Part model, mm, in its own coordinate system. A direction names the side the tool comes from. Give positions to 0.01 mm unless a question says otherwise; leave off trailing zeros. Loops run counter-clockwise (first coordinate to the right, second up) from the corner with the lowest first, then second, coordinate; pieces in that order, holes last. Notation, with made-up numbers: M 12,42 L 26,42 A27 cw 26,61 Z; hole C 20,-17.75 d8. An arc over 180 degrees is marked long. Answer in a Markdown table with one row per item.
from build123d import *

# Parameters (mm, degrees)
SKETCH1_R           = 2.5
BOSS_EXTRUDE1_DEPTH = 2.5


with BuildPart() as part:
    # Sketch1 → Boss-Extrude1 (new body)
    with BuildSketch(Plane(origin=(0, 0, -1.25), x_dir=(-1, 0, 0), z_dir=(0, 0, -1))):
        with BuildLine():
            Line((44.196, 6.35), (13.62993597, 36.91606403))
            ThreePointArc((13.62993597, 36.91606403), (12.941682484, 37.946108163), (12.7, 39.161128061))
            Line((12.7, 39.161128061), (12.7, 50.546))
            Line((12.7, 50.546), (6.35, 56.896))
            Line((6.35, 56.896), (-6.35, 56.896))
            Line((-6.35, 56.896), (-12.7, 50.546))
            Line((-12.7, 50.546), (-12.7, 39.161128061))
            ThreePointArc((-12.7, 39.161128061), (-12.941682484, 37.946108163), (-13.62993597, 36.91606403))
            Line((-13.62993597, 36.91606403), (-44.196, 6.35))
            Line((-44.196, 6.35), (-44.196, -6.35))
            Line((-44.196, -6.35), (-37.846, -12.7))
            Line((-37.846, -12.7), (37.846, -12.7))
            Line((37.846, -12.7), (44.196, -6.35))
            Line((44.196, -6.35), (44.196, 6.35))
        make_face()
        with Locations((0, 50.8)):
            Circle(SKETCH1_R, mode=Mode.SUBTRACT)
        with Locations((0, 38.1)):
            Circle(SKETCH1_R, mode=Mode.SUBTRACT)
        with Locations((-38.1, 0)):
            Circle(SKETCH1_R, mode=Mode.SUBTRACT)
        with Locations((-25.4, 0)):
            Circle(SKETCH1_R, mode=Mode.SUBTRACT)
        with Locations((-12.7, 0)):
            Circle(SKETCH1_R, mode=Mode.SUBTRACT)
        Circle(SKETCH1_R, mode=Mode.SUBTRACT)
        with Locations((12.7, 0)):
            Circle(SKETCH1_R, mode=Mode.SUBTRACT)
        with Locations((38.1, 0)):
            Circle(SKETCH1_R, mode=Mode.SUBTRACT)
        with Locations((25.4, 0)):
            Circle(SKETCH1_R, mode=Mode.SUBTRACT)
        with Locations((0, 12.7)):
            Circle(SKETCH1_R, mode=Mode.SUBTRACT)
        with Locations((0, 25.4)):
            Circle(SKETCH1_R, mode=Mode.SUBTRACT)
        with Locations((25.4, 12.7)):
            Circle(SKETCH1_R, mode=Mode.SUBTRACT)
        with Locations((12.7, 12.7)):
            Circle(SKETCH1_R, mode=Mode.SUBTRACT)
        with Locations((12.7, 25.4)):
            Circle(SKETCH1_R, mode=Mode.SUBTRACT)
        with Locations((-12.7, 12.7)):
            Circle(SKETCH1_R, mode=Mode.SUBTRACT)
        with Locations((-12.7, 25.4)):
            Circle(SKETCH1_R, mode=Mode.SUBTRACT)
        with Locations((-25.4, 12.7)):
            Circle(SKETCH1_R, mode=Mode.SUBTRACT)
    extrude(amount=-BOSS_EXTRUDE1_DEPTH)


solid = part.part
(1) Saw through at B-B (y = -1.5). Give the number of separate pieces and of enclosed holes in the cut face, plus the area to 3 significant figures.
Recorded:
| item | result |
|---|---|
| separate pieces | 8 |
| enclosed holes | 0 |
| area | 151 mm^2 |
(2) Saw through at D-D (y = 38.1). Write the cut outline in (x, z), plus the area to 3 significant figures.
Recorded:
| item | result |
|---|---|
| outline | M -12.88,-1.25 L -2.5,-1.25 L -2.5,1.25 L -12.88,1.25 Z; M 2.5,-1.25 L 12.88,-1.25 L 12.88,1.25 L 2.5,1.25 Z |
| area | 51.9 mm^2 |
(3) Saw through at A-A (y = 12.7). Write the cut outline in (x, z), plus the area to 3 significant figures.
Recorded:
| item | result |
|---|---|
| outline | M -37.85,-1.25 L -27.9,-1.25 L -27.9,1.25 L -37.85,1.25 Z; M -22.9,-1.25 L -15.2,-1.25 L -15.2,1.25 L -22.9,1.25 Z; M -10.2,-1.25 L -2.5,-1.25 L -2.5,1.25 L -10.2,1.25 Z; M 2.5,-1.25 L 10.2,-1.25 L 10.2,1.25 L 2.5,1.25 Z; M 15.2,-1.25 L 22.9,-1.25 L 22.9,1.25 L 15.2,1.25 Z; M 27.9,-1.25 L 37.85,-1.25 L 37.85,1.25 L 27.9,1.25 Z |
| area | 127 mm^2 |
(4) Pull direction X, two halves, no side cores. Call faces 3 (the face through (44.196, 0, 0)), 4 (the face through (1, 7, -1.25)), 5 (the face through (15.2, 0.1, 0)): +X half, -X half, draft (parallel to the pull), parting line (faces both ways), or undercut.
Recorded:
| item | result |
|---|---|
| face 3 | +X half |
| face 4 | draft |
| face 5 | undercut |
(5) Which spindle directions (+Z, -Z, +X, -X, +Y, -Y) get a long thin tool onto all of the face, cutting with end or side? Do faces 1 (the face through (-12.7, 45, 0)), 2 (the face through (0, 56.896, 0)). Say none if no direction does.
Recorded:
| item | result |
|---|---|
| face 1 | +Z, -Z, -X, +Y |
| face 2 | +Z, -Z, +X, -X, +Y |
(6) Drill centre lines: line 1 along Y through (x, z) = (0, 0); line 2 along Y through (x, z) = (-24, -1.05); line 3 along X through (y, z) = (12, -1). Where is each one in solid material? Low to high.
Recorded:
| item | result |
|---|---|
| line 1 | y = -12.7 to -2.5, 2.5 to 10.2, 15.2 to 22.9, 27.9 to 35.6, 40.6 to 48.3, 53.3 to 56.9 |
| line 2 | y = -12.7 to -2.07, 2.07 to 10.63, 14.77 to 26.55 |
| line 3 | x = -38.55 to -27.8, -23 to -15.1, -10.3 to -2.4, 2.4 to 10.3, 15.1 to 23, 27.8 to 38.55 |
